Job drawing, mm, ordinate dimensions from the low corner. One solid piece. A direction names the side the tool comes from. Round coordinates to 2 decimals unless told otherwise and drop trailing zeros. Write each loop counter-clockwise with the first axis right and the second up, starting at its lowest first coordinate (ties: lowest second). Pieces come first, ordered by that corner, then holes. Notation, with made-up numbers: (12, 25) -> (38, 25) arc R35 cw to (38, 63) -> close; hole circle Ø8 at (-6.75, 89.25). An arc over 180 degrees is marked (long way). Use CSV: the item, a comma, the result in double quotes. Start each with the question number.
(1) Probe line 1 (X direction, y = 13.25, z = 24.75); line 2 (Z direction, x = 18, y = 13). List the from-to ranges inside material, lowest first. Write a range as [from, to].
(2) Saw through at A-A (x = 20.75). Give the cut face in (y, z), plus the area to 3 significant figures.
(3) Saw through at D-D (y = 18.5). Give the cut face in (x, z).
(4) Two-plate mould, pull along X, no slides. Class the marked faces 3, 4, 5 and 6: released by +X, released by -X, zero draft, split by the parting line, or undercut.
(5) Saw through at C-C (x = 5.25). Give the cut face in (y, z), plus the area to 3 significant figures.
(6) Which spindle directions (+Z, -Z, +X, -X, +Y, -Y) get a long thin tool onto all of the face, cutting with end or side? Do the marked faces 1 and 2. Say none if no direction does.
(7) Drop flat-ended pins along their axis: pin 1 (8 mm diameter, centred on y = 13, z = 13, fed in from -X); pin 2 (1 mm diameter, centred on x = 17, y = 18, fed in from -Z); pin 3 (5 mm diameter, centred on x = 16, y = 15.5, fed in from +Z); pin 4 (1.5 mm diameter, centred on y = 12, z = 12.5, fed in from +X). Give the stop position or say it passes through.
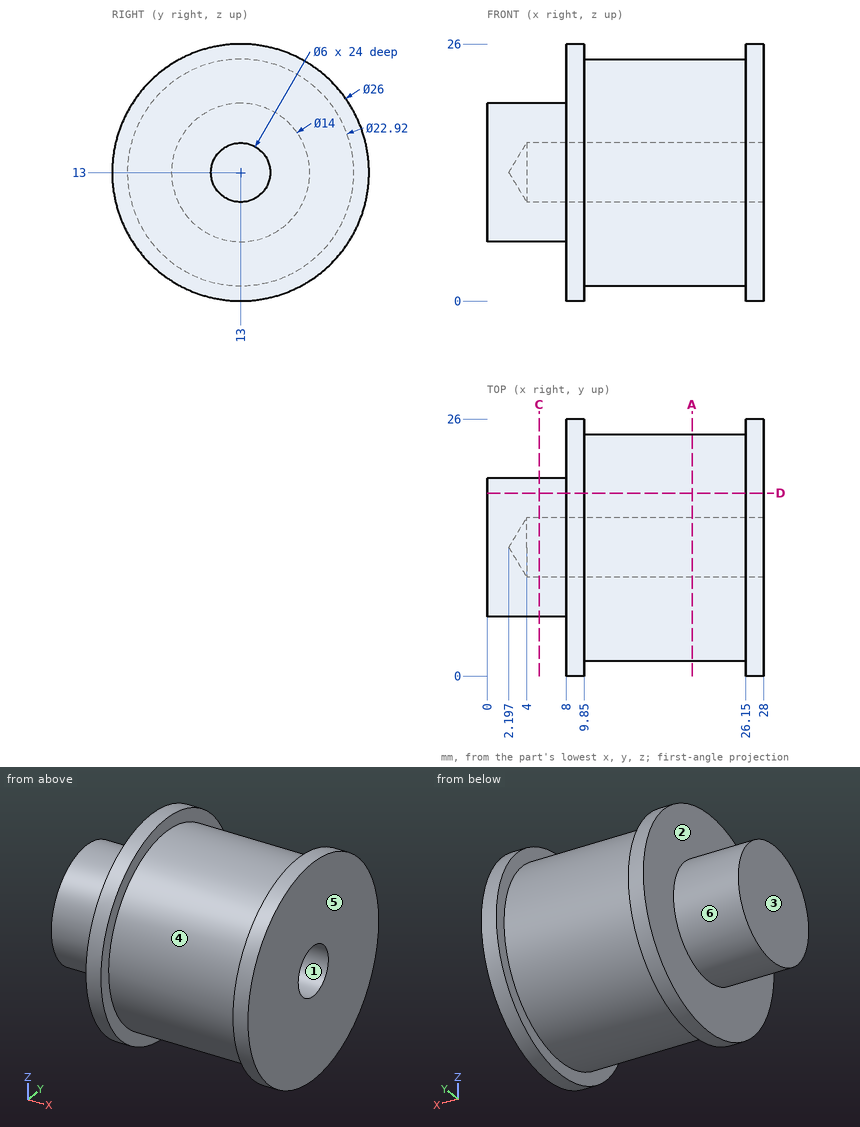
Answers:
1,line 1,"x = [8, 9.85], [26.15, 28]"
1,line 2,"z = [1.54, 10], [16, 24.46]"
2,outline,"circle Ø22.92 at (13, 13); hole circle Ø6 at (13, 13)"
2,area,"384 mm²"
3,outline,"(0, 8.67) -> (8, 8.67) -> (8, 1.22) -> (9.85, 1.22) -> (9.85, 2.95) -> (26.15, 2.95) -> (26.15, 1.22) -> (28, 1.22) -> (28, 24.78) -> (26.15, 24.78) -> (26.15, 23.05) -> (9.85, 23.05) -> (9.85, 24.78) -> (8, 24.78) -> (8, 17.33) -> (0, 17.33) -> close"
4,face 3,"released by -X"
4,face 4,"undercut"
4,face 5,"released by +X"
4,face 6,"zero draft"
5,outline,"circle Ø14 at (13, 13); hole circle Ø6 at (13, 13)"
5,area,"126 mm²"
6,face 1,"+X"
6,face 2,"-X"
7,pin 1,"stops at x = 0"
7,pin 2,"stops at z = 2.46"
7,pin 3,"stops at z = 24.46"
7,pin 4,"stops at x = 3.32"
